from build123d import *

# Parameters (mm, degrees)
SZKIC3_R                    = 1.10000034
DODANIE_WYCI_GNI_CIE2_DEPTH = 2
SZKIC7_R                    = 1.15000024
DODANIE_WYCI_GNI_CIE4_DEPTH = 2
ZAOKR_GLENIE1_R             = 1


with BuildPart() as part:
    # Szkic3 → Dodanie-wyciągnięcie2 (new body)
    with BuildSketch(Plane(origin=(38.160641903, 20.207828477, 157.30929901), x_dir=(0.972253346903095, -0.029805597670841302, -0.23202382589556209), z_dir=(0.23393039442477367, 0.12387698555880203, 0.964329333274237))):
        Polygon((-69.666310572, -102.553561212), (-79.264860968, -94.782442078), (-80.819178513, -93.5240451), (-77.043735552, -88.860781173), (-75.489418007, -90.119178151), (-65.890867611, -97.890297285), (-52.950125678, -108.367300905), (-56.725568639, -113.030564831), align=None)
        with Locations(Location((-57.169345947, -108.811046896, 0), (0, 0, 1.721249632))):
            Circle(SZKIC3_R, mode=Mode.SUBTRACT)
        with Locations(Location((-76.599691895, -93.079970126, 0), (0, 0, 1.721249632))):
            Circle(SZKIC3_R, mode=Mode.SUBTRACT)
    extrude(amount=DODANIE_WYCI_GNI_CIE2_DEPTH)

    # Szkic7 → Dodanie-wyciągnięcie4 (add)
    with BuildSketch(Plane(origin=(38.628502692, 20.455582448, 159.237957676), x_dir=(0.9722533469030947, -0.029805597670841396, -0.23202382589556286), z_dir=(0.23393039442477445, 0.12387698555880199, 0.9643293332742368))):
        with BuildLine():
            Line((-80.819178513, -93.5240451), (-175.638878356, -16.756704897))
            Line((-175.638878356, -16.756704897), (-194.757445315, -16.460528815))
            ThreePointArc((-194.757445315, -16.460528815), (-196.438982344, -17.373715152), (-198.273708049, -16.830338985))
            Line((-198.273708049, -16.830338985), (-199.491256389, -17.388602921))
            Line((-199.491256389, -17.388602921), (-198.273726955, -14.349785721))
            Line((-198.273726955, -14.349785721), (-195.616721108, -11.132918291))
            Line((-195.616721108, -11.132918291), (-195.127524487, -12.944294382))
            Line((-195.127524487, -12.944294382), (-181.856563591, -11.72278095))
            Line((-181.856563591, -11.72278095), (-178.08112063, -7.059517023))
            Line((-178.08112063, -7.059517023), (-179.648209308, 6.175086532))
            Line((-179.648209308, 6.175086532), (-181.521733094, 6.276601555))
            Line((-181.521733094, 6.276601555), (-178.718962553, 10.061139804))
            Line((-178.718962553, 10.061139804), (-176.20935813, 11.368191294))
            Line((-176.20935813, 11.368191294), (-176.502006841, 10.061139804))
            ThreePointArc((-176.502006841, 10.061139804), (-175.588684843, 8.379653584), (-176.131934764, 6.544869536))
            Line((-176.131934764, 6.544869536), (-171.863435395, -12.093440971))
            Line((-171.863435395, -12.093440971), (-77.043735552, -88.860781173))
            Line((-77.043735552, -88.860781173), (-80.819178513, -93.5240451))
        make_face()
        with Locations(Location((-178.074960694, 8.117983918, 0), (0, 0, 1.721249632))):
            Circle(SZKIC7_R, mode=Mode.SUBTRACT)
        with Locations(Location((-196.700467622, -14.887437029, 0), (0, 0, 1.721249632))):
            Circle(SZKIC7_R, mode=Mode.SUBTRACT)
    extrude(amount=-DODANIE_WYCI_GNI_CIE4_DEPTH)

    # Zaokrąglenie1
    # the kernel refuses this fillet: 1 mm, written as the material it adds along each edge
    with BuildSketch(Plane(origin=(-132.136984635, 9.070469004, 202.125371666), x_dir=(0.7556456600365923, -0.6472773151749931, -0.10015844311747091), z_dir=(-0.23393039442477445, -0.12387698555880199, -0.9643293332742368))) as zaokr_glenie1_piece_1:
        with BuildLine():
            CenterArc((ZAOKR_GLENIE1_R * 0.345368312497, ZAOKR_GLENIE1_R), ZAOKR_GLENIE1_R, 231.893419256, 38.106580745)
            Line((-ZAOKR_GLENIE1_R * 0.271757942514, ZAOKR_GLENIE1_R * 0.213135853291), (0, 0))
            Line((0, 0), (ZAOKR_GLENIE1_R * 0.345368312498, 0))
        make_face()
    extrude(amount=2)
    with BuildSketch(Plane(origin=(-128.466297581, 13.583197282, 200.655222001), x_dir=(0.755645659983129, -0.6472773152407205, -0.10015844309605833), z_dir=(-0.23393039442477445, -0.12387698555880199, -0.9643293332742368))) as zaokr_glenie1_piece_2:
        with BuildLine():
            CenterArc((ZAOKR_GLENIE1_R * 0.345368517806, -ZAOKR_GLENIE1_R), ZAOKR_GLENIE1_R, 89.999999995, 38.106601769)
            Line((-ZAOKR_GLENIE1_R * 0.271758025873, -ZAOKR_GLENIE1_R * 0.213136079689), (0, 0))
            Line((0, 0), (ZAOKR_GLENIE1_R * 0.345368517893, 0))
        make_face()
    extrude(amount=2)
    # the kernel refuses this fillet: 1 mm, written as the material it takes off along each edge
    with BuildSketch(Plane(origin=(-150.430265808, 15.842388646, 210.703360527), x_dir=(-0.6191538304813691, -0.7457448210428924, 0.24599430092575822), z_dir=(-0.23393039442477445, -0.12387698555880199, -0.9643293332742368))) as zaokr_glenie1_2_piece_1:
        with BuildLine():
            CenterArc((1.932614717, -1), ZAOKR_GLENIE1_R, 90, 122.052914314)
            Line((1.085056378, -1.530702235), (0, 0))
            Line((0, 0), (1.932614717, 0))
        make_face()
    extrude(amount=11.663073583, mode=Mode.SUBTRACT)
    with BuildSketch(Plane(origin=(-154.176575818, 9.764143782, 212.484809281), x_dir=(0.8837805609022797, 0.3863007559342876, -0.2640144809207439), z_dir=(-0.23393039442477445, -0.12387698555880199, -0.9643293332742368))) as zaokr_glenie1_2_piece_2:
        with BuildLine():
            CenterArc((2.115550514, -0.630589135), ZAOKR_GLENIE1_R, 140.906398732, 85.559709417)
            Line((1.426766982, -1.355556201), (0, 0))
            Line((0, 0), (1.339433679, 0))
        make_face()
    extrude(amount=11.840219302, mode=Mode.SUBTRACT)
    with BuildSketch(Plane(origin=(-136.76997961, 32.666813554, 205.035015593), x_dir=(0.9708292594479915, -0.08342561993848581, -0.22479037999332602), z_dir=(-0.23393039442477445, -0.12387698555880199, -0.9643293332742368))) as zaokr_glenie1_2_piece_3:
        with BuildLine():
            CenterArc((ZAOKR_GLENIE1_R * 1.85804027171, -ZAOKR_GLENIE1_R), ZAOKR_GLENIE1_R, 90, 123.421594356)
            Line((ZAOKR_GLENIE1_R * 1.02339993985, -ZAOKR_GLENIE1_R * 1.55079534897), (0, 0))
            Line((0, 0), (ZAOKR_GLENIE1_R * 1.85804027171, 0))
        make_face()
    extrude(amount=11.290201359, mode=Mode.SUBTRACT)
    with BuildSketch(Plane(origin=(-131.602089653, 37.560111501, 203.16570616), x_dir=(-0.8623099936693889, -0.4317250154405725, 0.26464123990930793), z_dir=(-0.23393039442477445, -0.12387698555880199, -0.9643293332742368))) as zaokr_glenie1_2_piece_4:
        with BuildLine():
            CenterArc((1.863025718, -1), ZAOKR_GLENIE1_R, 90, 91.379076601)
            Line((0.863315373, -1.024067103), (0, 0))
            Line((0, 0), (1.863025718, 0))
        make_face()
    extrude(amount=11.315128591, mode=Mode.SUBTRACT)
    with BuildSketch(Plane(origin=(-13.905120992, -86.007744656, 180.991487948), x_dir=(-0.6117811757755813, -0.7521213796372446, 0.24502494415715118), z_dir=(0.23393039442477367, 0.12387698555880203, 0.964329333274237)), Plane(origin=(-17.575808047, -90.520472934, 182.461637613), x_dir=(-0.7556456600354768, 0.6472773151763643, 0.10015844311702354), z_dir=(0.23393039442477367, 0.12387698555880203, 0.964329333274237))) as zaokr_glenie1_2_piece_5:
        with BuildLine():
            CenterArc((ZAOKR_GLENIE1_R, -ZAOKR_GLENIE1_R), ZAOKR_GLENIE1_R, 90, 90)
            Line((0, -ZAOKR_GLENIE1_R), (0, 0))
            Line((0, 0), (ZAOKR_GLENIE1_R, 0))
        make_face()
    extrude(amount=7, mode=Mode.SUBTRACT)


solid = part.part
Check sheet for the modelled part. Datum: model origin and axes. Units: mm. A direction names the side the tool comes from. Round coordinates to 2 decimals unless told otherwise and drop trailing zeros. Loops run counter-clockwise (first coordinate to the right, second up) from the corner with the lowest first, then second, coordinate; pieces in that order, holes last. Notation, with made-up numbers: (15, 9.25) -> (69, 9.25) arc R14 cw to (69, 32.25) -> close; hole circle Ø1 at (66.25, 48). An arc over 180 degrees is marked (long way). Put each result on its own line as item: value. Start each with the question number.
1. Gauge pin test, flat ends, axial feed: pin 1 (1.5 mm diameter, centred on y = -45.5, z = 192, fed in from +X); pin 2 (8 mm diameter, centred on x = -85.5, z = 202.5, fed in from -Y); pin 3 (12 mm diameter, centred on x = -32, z = 186, fed in from -Y). Record the tip position at first contact, or that the pin passes through.
2. Section check B-B (y = -13). Enter the section's corners in (x, z).
3. Section check A-A (z = 195). Enter the section's corners in (x, y), plus the area to 3 significant figures.
4. Draft check along Y on faces 3 (the face through (-135.493, 25.134, 199.854)), 4 (the face through (-14.908, -87.811, 185.081)), 5 (the face through (-144.954, 13.713, 203.616)), 6 (the face through (-136.603, 16.351, 201.251)). Enter one of: +Y half, -Y half, draft (parallel to the pull), parting line (faces both ways), or undercut.
5. Access from +Z, -Z, +X, -X, +Y, -Y to the whole of each face (thin tool, end or side, straight path). Record for faces 1 (the face through (-84.321, -28.119, 195.303)), 2 (the face through (-130.838, 23.064, 198.99)).
6. Scan line: probe 1 along Z at (x, y) = (-73, -40). Record every from-to range of solid material in increasing order.
Findings:
1. pin 1: stops at x = -58.91
1. pin 2: passes through
1. pin 3: stops at y = -82.49
2. outline: (-107.13, 196.82) -> (-98.19, 194.65) -> (-97.43, 196.54) -> (-106.37, 198.71) -> close
3. outline: (-100.82, -10.75) -> (-93.4, -24.76) -> (-78.38, -36.98) -> (-85.8, -22.96) -> close
3. area: 120 mm^2
4. face 3: undercut
4. face 4: -Y half
4. face 5: +Y half
4. face 6: undercut
5. face 1: +Z, +X, +Y
5. face 2: -Z, +X
6. probe 1: z = 192.01 to 194.08
